from build123d import *

# Parameters (mm, degrees)
SKETCH1_W           = 1803.4
SKETCH1_H           = 558.8
BOSS_EXTRUDE1_DEPTH = 2133.6
SHELL1_T            = -2.54


with BuildPart() as part:
    # Sketch1 → Boss-Extrude1 (new body)
    with BuildSketch(Plane(origin=(0, 0, 0), x_dir=(1, 0, 0), z_dir=(0, 1, 0))):
        Rectangle(SKETCH1_W, SKETCH1_H)
    extrude(amount=BOSS_EXTRUDE1_DEPTH)

    # Shell1
    shell1_openings = [part.faces().sort_by_distance(p)[0] for p in [
        (0, 1066.8, 279.4),
    ]]
    offset(amount=SHELL1_T, openings=shell1_openings, kind=Kind.INTERSECTION)


solid = part.part
The model under review builds one solid part; all positions refer to its coordinate system, in mm. A direction names the side the tool comes from. Coordinates: 2 decimals unless noted, no trailing zeros. Write each loop counter-clockwise with the first axis right and the second up, starting at its lowest first coordinate (ties: lowest second). Pieces come first, ordered by that corner, then holes. Notation, with made-up numbers: (22.25, -8.5) - (62.25, -8.5) arc R21 cw to (62.25, 18.5) - close; hole circle Ø1 at (84, 56). An arc over 180 degrees is marked (long way). Answer as a JSON object with one key per item and string values. Group by question number.
1. To check wall thickness, follow probe 1 along X at (y, z) = (429, 114.5); probe 2 along Y at (x, z) = (174, 14); probe 3 along Z at (x, y) = (648.5, 689.5). State the ranges of each line that lie inside material, in increasing order.
2. Mouldability with a two-part tool opening along Y and no side actions: class faces 3 (the face through (-13, 2133.6, -4)), 4 (the face through (-13, 2.54, -3)), 5 (the face through (-899.16, 1052, 5)), 6 (the face through (-13, 1052, -279.4)) as pulls with the +Y half, pulls with the -Y half, needs draft (parallel to the pull), parting line crosses it, or undercut.
3. Add section A-A (z = -7.5). Give the boundary of the cut face in (x, y).
4. Machinability: for faces 1 (the face through (-901.7, 1052, 4)), 2 (the face through (899.16, 1052, 5)), which of the approach directions +Z, -Z, +X, -X, +Y, -Y give a long, thin tool a straight path to every point of the face, cutting with its end or side? Answer none if there is none.
5. Add section B-B (y = 1663). Give the boundary of the cut face in (x, z).
6. Clearance check with a flat-ended pin moving along its axis: pin 1 Ø1 at (x, y) = (121.5, 1140) entering from +Z. State where the tip first meets the part, or that it passes through.
7. Add section C-C (x = 345). Give the boundary of the cut face in (y, z).
Findings:
{
 "1": {"probe 1": "-901.7 to -899.16, 899.16 to 901.7", "probe 2": "0 to 2.54, 2131.06 to 2133.6", "probe 3": "-279.4 to -276.86"},
 "2": {"face 3": "pulls with the +Y half", "face 4": "undercut", "face 5": "undercut", "face 6": "needs draft"},
 "3": {"outline": "(-901.7, 0) - (901.7, 0) - (901.7, 2133.6) - (-901.7, 2133.6) - close; hole (-899.16, 2.54) - (899.16, 2.54) - (899.16, 2131.06) - (-899.16, 2131.06) - close"},
 "4": {"face 1": "+Z, -Z, -X, +Y, -Y", "face 2": "+Z"},
 "5": {"outline": "(-901.7, -279.4) - (901.7, -279.4) - (901.7, 279.4) - (899.16, 279.4) - (899.16, -276.86) - (-899.16, -276.86) - (-899.16, 279.4) - (-901.7, 279.4) - close"},
 "6": {"pin 1": "z = -276.86"},
 "7": {"outline": "(0, -279.4) - (2133.6, -279.4) - (2133.6, 279.4) - (2131.06, 279.4) - (2131.06, -276.86) - (2.54, -276.86) - (2.54, 279.4) - (0, 279.4) - close"}
}
